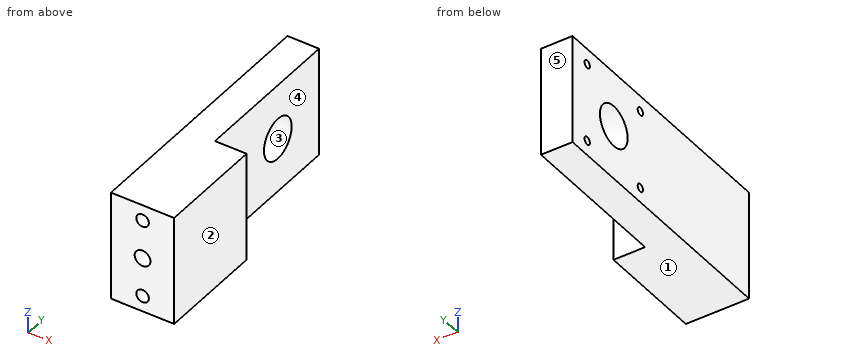
```python
from build123d import *

# Parameters (mm, degrees)
SKETCH1_W                 = 20
SKETCH1_H                 = 34.7
BOSS_EXTRUDE1_DEPTH       = 83
CUT_EXTRUDE2_REACH        = 36.7
SKETCH3_W                 = 10
SKETCH3_H                 = 48.965000852
CUT_EXTRUDE3_REACH        = 22
SKETCH4_R                 = 6.5
M3X0_5_TAPPED_HOLE1_D     = 2.5
M3X0_5_TAPPED_HOLE1_DEPTH = 7.5
M3X0_5_TAPPED_HOLE1_TIP   = 0.751075774
M6X1_0_TAPPED_HOLE1_D     = 5
M6X1_0_TAPPED_HOLE1_DEPTH = 15
M6X1_0_TAPPED_HOLE1_TIP   = 1.502151548
F_4_0MM_DOWEL_HOLE1_D     = 4
F_4_0MM_DOWEL_HOLE1_DEPTH = 5.2
F_4_0MM_DOWEL_HOLE1_TIP   = 1.201721238


with BuildPart() as part:
    # Sketch1 → Boss-Extrude1 (new body)
    with BuildSketch(Plane(origin=(0, 0, 0), x_dir=(1, 0, 0), z_dir=(0, 1, 0))):
        with Locations((5.656892123, -5.553125)):
            Rectangle(SKETCH1_W, SKETCH1_H)
    extrude(amount=BOSS_EXTRUDE1_DEPTH)

    # Sketch3 → Cut-Extrude2 (cut, up to next)
    with BuildSketch(Plane(origin=(0, 0, -11.796875), x_dir=(-1, 0, 0), z_dir=(0, 0, -1)), mode=Mode.PRIVATE) as cut_extrude2_sk1:
        with Locations((-10.656892123, 58.517499574)):
            Rectangle(SKETCH3_W, SKETCH3_H)
    cut_extrude2_tool1 = extrude(cut_extrude2_sk1.sketch, amount=-CUT_EXTRUDE2_REACH, mode=Mode.PRIVATE) & part.part
    add(cut_extrude2_tool1.solids().sort_by_distance((10.656892, 58.5175, -11.796875))[0], mode=Mode.SUBTRACT)

    # Sketch4 → Cut-Extrude3 (cut, up to next)
    with BuildSketch(Plane.ZY.offset(4.343107877), mode=Mode.PRIVATE) as cut_extrude3_sk1:
        with Locations((5.403125, 63.609645263)):
            Circle(SKETCH4_R)
    cut_extrude3_tool1 = extrude(cut_extrude3_sk1.sketch, amount=-CUT_EXTRUDE3_REACH, mode=Mode.PRIVATE) & part.part
    add(cut_extrude3_tool1.solids().sort_by_distance((-4.343108, 63.609645, 5.403125))[0], mode=Mode.SUBTRACT)

    # M3x0.5 Tapped Hole1
    with Locations(Plane.ZY.offset(4.343107877)):
        with Locations((-7.096875, 51.109645263), (17.903125, 51.109645263), (17.903125, 76.109645263), (-7.096875, 76.109645263)):
            Hole(M3X0_5_TAPPED_HOLE1_D / 2, depth=M3X0_5_TAPPED_HOLE1_DEPTH)
            with Locations((0, 0, -(M3X0_5_TAPPED_HOLE1_DEPTH + M3X0_5_TAPPED_HOLE1_TIP / 2))):  # 118° drill point
                Cone(0, M3X0_5_TAPPED_HOLE1_D / 2, M3X0_5_TAPPED_HOLE1_TIP, mode=Mode.SUBTRACT)

    # M6x1.0 Tapped Hole1
    with Locations(Plane(origin=(0, 0, 0), x_dir=(-1, 0, 0), z_dir=(0, -1, 0))):
        with Locations((-5.656892123, -5.553125)):
            Hole(M6X1_0_TAPPED_HOLE1_D / 2, depth=M6X1_0_TAPPED_HOLE1_DEPTH)
            with Locations((0, 0, -(M6X1_0_TAPPED_HOLE1_DEPTH + M6X1_0_TAPPED_HOLE1_TIP / 2))):  # 118° drill point
                Cone(0, M6X1_0_TAPPED_HOLE1_D / 2, M6X1_0_TAPPED_HOLE1_TIP, mode=Mode.SUBTRACT)

    # Ø4.0mm Dowel Hole1
    with Locations(Plane(origin=(0, 0, 0), x_dir=(-1, 0, 0), z_dir=(0, -1, 0))):
        with Locations((-5.656892123, -17.903125), (-5.656892123, 6.796875)):
            Hole(F_4_0MM_DOWEL_HOLE1_D / 2, depth=F_4_0MM_DOWEL_HOLE1_DEPTH)
            with Locations((0, 0, -(F_4_0MM_DOWEL_HOLE1_DEPTH + F_4_0MM_DOWEL_HOLE1_TIP / 2))):  # 118° drill point
                Cone(0, F_4_0MM_DOWEL_HOLE1_D / 2, F_4_0MM_DOWEL_HOLE1_TIP, mode=Mode.SUBTRACT)


solid = part.part
```
Input: part model. Units: mm. Frame: model coordinates. Face numbers are marked on the shaded views. A direction names the side the tool comes from. Give positions to 0.01 mm unless a question says otherwise; leave off trailing zeros. Order: outer loops, then holes, each group sorted by start corner. A loop starts at its lowest first (then second) coordinate and runs counter-clockwise, first axis right, second up. Notation, with made-up numbers: M 23.5,44 L 43.5,44 A18 cw 43.5,78 Z; hole C -8,54.5 d5. An arc over 180 degrees is marked long. Return JSON: item names as keys, results as strings.
1) Section query C-C on z = -3. Output: boundary loops of the cut face in (x, y) (3 decimals).
Taken from the geometry:
{"outline": "M -4.343,0 L 15.657,0 L 15.657,34.035 L 5.657,34.035 L 5.657,83 L -4.343,83 Z"}
2) Contact query for flat-ended pins moving along their axis: pin 1 (11 mm diameter, centred on x = 12.5, z = 7.5, fed in from +Y) (3 decimals); pin 2 (2 mm diameter, centred on y = 51.11, z = 17.9, fed in from -X); pin 3 (1.5 mm diameter, centred on y = 64, z = 9.5, fed in from -X); pin 4 (6.5 mm diameter, centred on x = 5.66, z = -6.8, fed in from -Y). Output: stop coordinate, or through.
Taken from the geometry:
{"pin 1": "stops at y = 34.035", "pin 2": "stops at x = 3.31", "pin 3": "passes through", "pin 4": "stops at y = 0"}
3) Line query: L1, parallel to X at y = 3.5, z = 5.5; L2, parallel to X at y = 42.5, z = -2.5; L3, parallel to Y at x = 14, z = -6 (3 decimals). Output: solid intervals per line, ascending. Write a range as [from, to].
Taken from the geometry:
{"L1": "x = [-4.34, 3.16], [8.16, 15.66]", "L2": "x = [-4.34, 5.66]", "L3": "y = [0, 34.035]"}
4) Access query for the marked faces 4 and 5. Directions: +Z, -Z, +X, -X, +Y, -Y. A direction counts if a zero-diameter tool reaches every point of the face in a straight line with its end or side. Return the directions, or none.
Taken from the geometry:
{"face 4": "+Z, -Z, +X, +Y", "face 5": "+Z, -Z, +X, -X, +Y"}
5) Mould query, pull axis Z, two halves, no side actions, for the marked faces 1, 2 and 3. Classes: released by +Z, released by -Z, zero draft, split by the parting line, or undercut.
Taken from the geometry:
{"face 1": "released by -Z", "face 2": "zero draft", "face 3": "undercut"}
6) Section query D-D on x = 0. Output: boundary loops of the cut face in (y, z).
Taken from the geometry:
{"outline": "M 0,-11.8 L 83,-11.8 L 83,22.9 L 0,22.9 Z; hole C 51.11,-7.1 d2.5; hole C 51.11,17.9 d2.5; hole C 63.61,5.4 d13; hole C 76.11,-7.1 d2.5; hole C 76.11,17.9 d2.5"}
7) Section query A-A on z = 10.5. Output: boundary loops of the cut face in (x, y) (3 decimals), and give its area (3 significant figures).
Taken from the geometry:
{"outline": "M -4.343,0 L 15.657,0 L 15.657,34.035 L 5.657,34.035 L 5.657,59.576 L -4.343,59.576 Z; M -4.343,67.643 L 5.657,67.643 L 5.657,83 L -4.343,83 Z", "area": "1,090 mm2"}
8) Section query B-B on y = 7.5. Output: boundary loops of the cut face in (x, z).
Taken from the geometry:
{"outline": "M -4.34,-11.8 L 15.66,-11.8 L 15.66,22.9 L -4.34,22.9 Z; hole C 5.66,5.55 d5"}
